```python
from build123d import *

# Parameters (mm, degrees)
F0_W           = 609.6
F0_H           = 38.1
F1_DEPTH       = 4.8133
F3_D           = 10.0838
F3_CSINK_D     = 19.8374
F3_CSINK_ANGLE = 82


with BuildPart() as f1:
    # F0 (on Top) → F1 (new body, symmetric)
    with BuildSketch(Plane.XY):
        Rectangle(F0_W, F0_H)
    extrude(amount=F1_DEPTH, both=True)

    # F3 (through all)
    with Locations(Plane.XY.offset(4.8133)):
        with Locations((-266.7, 0), (-88.9, 0), (88.9, 0), (266.7, 0)):
            CounterSinkHole(F3_D / 2, F3_CSINK_D / 2, counter_sink_angle=F3_CSINK_ANGLE)


solid = f1.part
```
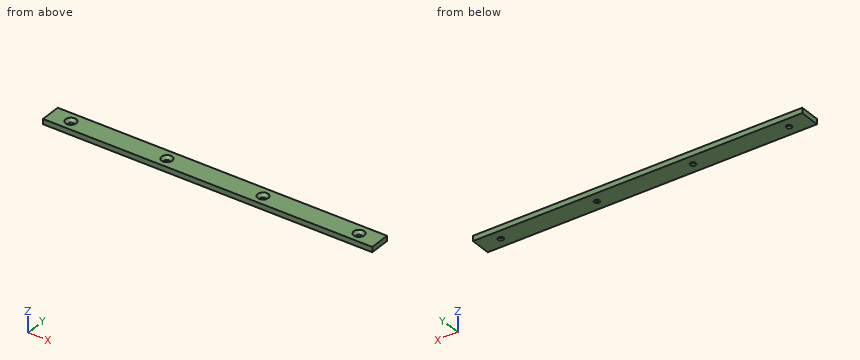
For this review, take the finished solid that the model builds, in its own axes (mm). Round coordinates to 2 decimals unless told otherwise and drop trailing zeros. Write each loop counter-clockwise with the first axis right and the second up, starting at its lowest first coordinate (ties: lowest second). Pieces come first, ordered by that corner, then holes. Notation, with made-up numbers: (-10, -18) -> (47, -18) arc R6 ccw to (47, -11) -> close; hole circle Ø7 at (70.5, 0). An arc over 180 degrees is marked (long way). Use one line per item in the form item = value.
1) Take a section at A-A, the plane x = 88.9. Write out the cut boundary in (y, z), and give its area (3 significant figures).
Found:
outline = (-19.05, -4.81) -> (-5.04, -4.81) -> (-5.04, -0.8) -> (-9.92, 4.81) -> (-19.05, 4.81) -> close; (5.04, -4.81) -> (19.05, -4.81) -> (19.05, 4.81) -> (9.92, 4.81) -> (5.04, -0.8) -> close
area = 242 mm2
2) Clearance check with a flat-ended pin moving along its axis: pin 1 (11.5 mm diameter, centred on x = -88.9, y = 0, fed in from -Z). State where the tip first meets the part, or that it passes through.
Found:
pin_1 = -4.81
3) To check wall thickness, follow L1, parallel to X at y = 0, z = -2.1; L2, parallel to Y at x = -90, z = -1.5; L3, parallel to X at y = -2.5, z = -4.5. State the ranges of each line that lie inside material, in increasing order. Write a range as from..to.
Found:
L1 = -304.8..-271.74, -261.66..-93.94, -83.86..83.86, 93.94..261.66, 271.74..304.8
L2 = -19.05..-4.92, 4.92..19.05
L3 = -304.8..-271.08, -262.32..-93.28, -84.52..84.52, 93.28..262.32, 271.08..304.8
4) Take a section at B-B, the plane z = 1. Write out the cut boundary in (x, y), and give its area (3 significant figures).
Found:
outline = (-304.8, -19.05) -> (304.8, -19.05) -> (304.8, 19.05) -> (-304.8, 19.05) -> close; hole circle Ø13.21 at (-266.7, 0); hole circle Ø13.21 at (-88.9, 0); hole circle Ø13.21 at (88.9, 0); hole circle Ø13.21 at (266.7, 0)
area = 22,700 mm2
